from build123d import *

# Parameters (mm, degrees)
BOSS_EXTRUDE1_DEPTH        = 7.5
CUT_EXTRUDE1_DEPTH         = 1.5
SKETCH4_R                  = 3.5
CUT_EXTRUDE3_DEPTH         = 2.5
SKETCH5_R                  = 2.05
CUT_EXTRUDE4_DEPTH         = 38.414330746
F_3_1_3_1_DIAMETER_HOLE1_D = 3.1


with BuildPart() as part:
    # Sketch1 → Boss-Extrude1 (new body)
    with BuildSketch(Plane(origin=(0, 0, 0), x_dir=(1, 0, 0), z_dir=(0, 1, 0))):
        with BuildLine():
            Line((-199.423569985, 35.163755978), (-184.65145369, 32.559033313))
            ThreePointArc((-184.65145369, 32.559033313), (-187.5, 0), (-184.65145369, -32.559033313))
            Line((-184.65145369, -32.559033313), (-199.423569985, -35.163755978))
            ThreePointArc((-199.423569985, -35.163755978), (-202.5, 0), (-199.423569985, 35.163755978))
        make_face()
    extrude(amount=BOSS_EXTRUDE1_DEPTH)

    # Sketch2 → Cut-Extrude1 (cut)
    with BuildSketch(Plane(origin=(0, 7.5, 0), x_dir=(1, 0, 0), z_dir=(0, 1, 0))):
        with BuildLine():
            Line((-187.113473072, 32.993153757), (-196.961550602, 34.729635533))
            ThreePointArc((-196.961550602, 34.729635533), (-198.7407137, 22.408228804), (-199.749843554, 10))
            Line((-199.749843554, 10), (-189.73665961, 10))
            ThreePointArc((-189.73665961, 10), (-188.775466906, 21.536552519), (-187.113473072, 32.993153757))
        make_face()
        with BuildLine():
            Line((-189.73665961, -10), (-199.749843554, -10))
            ThreePointArc((-199.749843554, -10), (-198.7407137, -22.408228804), (-196.961550602, -34.729635533))
            Line((-196.961550602, -34.729635533), (-187.113473072, -32.993153757))
            ThreePointArc((-187.113473072, -32.993153757), (-188.775466906, -21.536552519), (-189.73665961, -10))
        make_face()
    extrude(amount=-CUT_EXTRUDE1_DEPTH, mode=Mode.SUBTRACT)

    # Sketch4 → Cut-Extrude3 (cut)
    with BuildSketch(Plane(origin=(-195, 0, 0), x_dir=(0, 0, -1), z_dir=(1, 0, 0))):
        with Locations((0, 7.5)):
            Circle(SKETCH4_R)
    extrude(amount=-CUT_EXTRUDE3_DEPTH, mode=Mode.SUBTRACT)

    # Sketch5 → Cut-Extrude4 (cut, through all)
    with BuildSketch(Plane(origin=(-195, 0, 0), x_dir=(0, 0, -1), z_dir=(1, 0, 0))):
        with Locations((0, 7.5)):
            Circle(SKETCH5_R)
    extrude(amount=CUT_EXTRUDE4_DEPTH, mode=Mode.SUBTRACT)

    # Ø3.1 (3.1) Diameter Hole1 (through all)
    with Locations(Plane(origin=(0, 0, 0), x_dir=(-1, 0, 0), z_dir=(0, -1, 0))):
        with Locations((194.257966128, -16.995369836), (194.257966128, 16.995369836)):
            Hole(F_3_1_3_1_DIAMETER_HOLE1_D / 2)


solid = part.part
The listing builds one solid part. Answer for the finished solid, in the listing's coordinates (mm). A direction names the side the tool comes from. Give positions to 0.01 mm unless a question says otherwise; leave off trailing zeros. Order: outer loops, then holes, each group sorted by start corner. A loop starts at its lowest first (then second) coordinate and runs counter-clockwise, first axis right, second up. Notation, with made-up numbers: (67, 22.25) -> (116, 22.25) arc R23 ccw to (116, 54.25) -> close; hole circle Ø6 at (74, 22). An arc over 180 degrees is marked (long way). Put each result on its own line as item: value.
Item 1: For a pull along Z with two mould halves and no side action, classify faces 4 (the face through (-187.5, 3.7, -0.5)), 5 (the face through (-195, 5, 0)), 6 (the face through (-193, 0, 0)), 7 (the face through (-188.757, 6.76, 21.698)) as released by +Z, released by -Z, zero draft, split by the parting line, or undercut.
Established:
face 4: undercut
face 5: undercut
face 6: zero draft
face 7: released by +Z
Item 2: A cutting plane is placed at B-B on x = -188.25. Give the vertices of the cut face in (y, z), plus the area to 3 significant figures.
Established:
outline: (0, -33.19) -> (6, -33.19) -> (6, -25.73) -> (7.5, -25.73) -> (7.5, -2.05) arc R2.05 cw to (7.5, 2.05) -> (7.5, 25.73) -> (6, 25.73) -> (6, 33.19) -> (0, 33.19) -> close
area: 469 mm^2
Item 3: For faces 1 (the face through (-188.794, 6.76, -21.375)), 2 (the face through (-192.14, 2.86, -33.88)), 3 (the face through (-194, 6, -23)), determine the directions among +Z, -Z, +X, -X, +Y, -Y from which every point of the face is accessible in a straight line to the end or side of a thin tool.
Established:
face 1: -Z, +Y
face 2: -Z, +X, +Y, -Y
face 3: +Y
Item 4: Straight lines are drawn through the part: line 1 (Z direction, x = -195.25, y = 3.75); line 2 (X direction, y = 6, z = -2); line 3 (Z direction, x = -194, y = 5). For each, find the intervals that lie inside material, in ascending order.
Established:
line 1: z = -34.43 to -18.19, -15.8 to 15.8, 18.19 to 34.43
line 2: x = -202.49 to -197.5, -195 to -187.49
line 3: z = -34.21 to -18.52, -15.47 to 15.47, 18.52 to 34.21
Item 5: A cutting plane is placed at C-C on y = 6.75. Give the vertices of the cut face in (x, z).
Established:
outline: (-199.75, -10) -> (-189.74, -10) arc R190 ccw to (-187.11, -32.99) -> (-184.65, -32.56) arc R187.5 cw to (-187.49, -1.91) -> (-195, -1.91) -> (-195, -3.42) -> (-197.5, -3.42) -> (-197.5, 3.42) -> (-195, 3.42) -> (-195, 1.91) -> (-187.49, 1.91) arc R187.5 cw to (-184.65, 32.56) -> (-187.11, 32.99) arc R190 ccw to (-189.74, 10) -> (-199.75, 10) arc R200 cw to (-196.96, 34.73) -> (-199.42, 35.16) arc R202.5 ccw to (-199.42, -35.16) -> (-196.96, -34.73) arc R200 cw to start
Item 6: Given P1, Ø1.2, axis at x = -194.5, y = 6.5, coming from the +Z side; P2, Ø3, axis at y = 2.5, z = 17.5, coming from the -X side; P3, Ø3, axis at y = 1.5, z = 25.5, coming from the -X side, each flat-ended and moving along its own axis, determine where each tip first touches the part or whether it passes through.
Established:
P1: stops at z = 34.35
P2: stops at x = -201.87
P3: stops at x = -201.07
Item 7: A cutting plane is placed at D-D on z = 23. Give the vertices of the cut face in (x, y), plus the area to 3 significant figures.
Established:
outline: (-201.19, 0) -> (-186.08, 0) -> (-186.08, 7.5) -> (-188.6, 7.5) -> (-188.6, 6) -> (-198.67, 6) -> (-198.67, 7.5) -> (-201.19, 7.5) -> close
area: 98.2 mm^2
Item 8: A cutting plane is placed at A-A on z = 0. Give the vertices of the cut face in (x, y), plus the area to 3 significant figures.
Established:
outline: (-202.5, 0) -> (-187.5, 0) -> (-187.5, 5.45) -> (-195, 5.45) -> (-195, 4) -> (-197.5, 4) -> (-197.5, 7.5) -> (-202.5, 7.5) -> close
area: 88.4 mm^2
